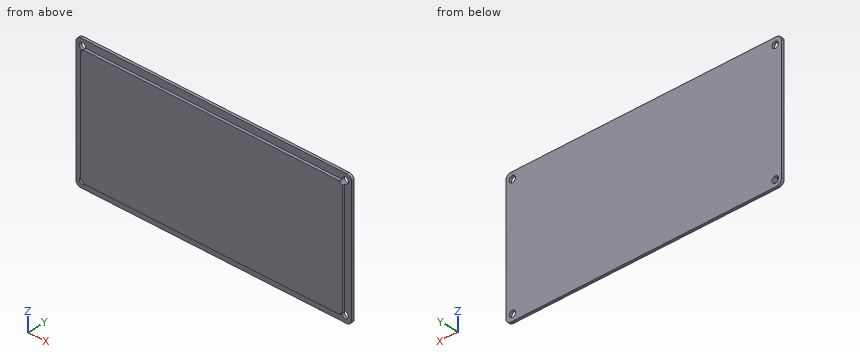
```python
from build123d import *

# Parameters (mm, degrees)
SKETCH2_W           = 127
SKETCH2_H           = 57.15
BOSS_EXTRUDE3_DEPTH = 1.27
SKETCH3_W           = 133.35
SKETCH3_H           = 63.5
BOSS_EXTRUDE4_DEPTH = 1.27
SKETCH4_R           = 1.524
CUT_EXTRUDE1_DEPTH  = 74.892284611
FILLET1_R           = 2.54
SKETCH5_W           = 127
SKETCH5_H           = 57.15
SKETCH5_W_2         = 126.5428
SKETCH5_H_2         = 56.6928
CUT_EXTRUDE2_DEPTH  = 1.27


with BuildPart() as part:
    # Sketch2 → Boss-Extrude3 (new body)
    with BuildSketch(Plane(origin=(0, 0, 0), x_dir=(1, 0, 0), z_dir=(0, 1, 0))):
        Rectangle(SKETCH2_W, SKETCH2_H)
    extrude(amount=BOSS_EXTRUDE3_DEPTH)

    # Sketch3 → Boss-Extrude4 (add)
    with BuildSketch(Plane(origin=(0, 1.27, 0), x_dir=(1, 0, 0), z_dir=(0, 1, 0))):
        Rectangle(SKETCH3_W, SKETCH3_H)
    extrude(amount=BOSS_EXTRUDE4_DEPTH)

    # Sketch4 → Cut-Extrude1 (cut, through all)
    with BuildSketch(Plane(origin=(0, 0, 0), x_dir=(-1, 0, 0), z_dir=(0, -1, 0))):
        with Locations(Location((63.5, -28.575, 0), (0, 0, 90))):
            Circle(SKETCH4_R)
        with Locations(Location((-63.5, -28.575, 0), (0, 0, 90))):
            Circle(SKETCH4_R)
        with Locations(Location((-63.5, 28.575, 0), (0, 0, 90))):
            Circle(SKETCH4_R)
        with Locations(Location((63.5, 28.575, 0), (0, 0, 90))):
            Circle(SKETCH4_R)
    extrude(amount=-CUT_EXTRUDE1_DEPTH, mode=Mode.SUBTRACT)

    # Fillet1
    fillet1_edges = [part.edges().sort_by_distance(p)[0] for p in [
        (66.675, 1.905, 31.75),
        (66.675, 1.905, -31.75),
        (-66.675, 1.905, -31.75),
        (-66.675, 1.905, 31.75),
    ]]
    fillet(fillet1_edges, radius=FILLET1_R)

    # Sketch5 → Cut-Extrude2 (cut)
    with BuildSketch(Plane(origin=(0, 0, 0), x_dir=(-1, 0, 0), z_dir=(0, -1, 0))):
        Rectangle(SKETCH5_W, SKETCH5_H)
        Rectangle(SKETCH5_W_2, SKETCH5_H_2, mode=Mode.SUBTRACT)
    extrude(amount=-CUT_EXTRUDE2_DEPTH, mode=Mode.SUBTRACT)


solid = part.part
```
Geometry: final body of the model. Coordinates: model frame, mm. Round coordinates to 2 decimals unless told otherwise and drop trailing zeros. Order: outer loops, then holes, each group sorted by start corner. A loop starts at its lowest first (then second) coordinate and runs counter-clockwise, first axis right, second up. Notation, with made-up numbers: (8, -33) - (59, -33) arc R22 ccw to (59, 3) - close; hole circle Ø2 at (-16, 61). An arc over 180 degrees is marked (long way). Use CSV: the item, a comma, the result in double quotes. Start each with the question number.
Q1. Section query A-A (z = 20). Return loops of the section in (x, y) (3 decimals).
Q2. First-contact query: pin 1 (1.4 mm diameter, centred on y = 0.5, z = 7.5, fed in from -X); pin 2 (1 mm diameter, centred on x = -30, y = 0.5, fed in from +Z); pin 3 (1 mm diameter, centred on x = 19.5, y = 0.5, fed in from -Z). Flat tips, straight axial feed; report the tip coordinate or a pass-through.
Q3. Section query B-B (y = 0.75). Return loops of the section in (x, z) (3 decimals), and give its area (3 significant figures).
Q4. Material intervals for line 1 along Z through (x, y) = (63.5, 1.3); line 2 along Z through (x, y) = (60, 1.2); line 3 along X through (y, z) = (0.75, -15), sorted ascending. Write a range as from..to.
Result set:
1,outline,"(-66.675, 1.27) - (-63.271, 1.27) - (-63.271, 0) - (63.271, 0) - (63.271, 1.27) - (66.675, 1.27) - (66.675, 2.54) - (-66.675, 2.54) - close"
2,pin 1,"stops at x = -63.27"
2,pin 2,"stops at z = 28.35"
2,pin 3,"stops at z = -28.35"
3,outline,"(-63.271, -27.068) arc R1.524 cw to (-61.993, -28.346) - (61.993, -28.346) arc R1.524 cw to (63.271, -27.068) - (63.271, 27.068) arc R1.524 cw to (61.993, 28.346) - (-61.993, 28.346) arc R1.524 cw to (-63.271, 27.068) - close"
3,area,"7,170 mm2"
4,line 1,"z = -31.75..-30.1, -27.05..27.05, 30.1..31.75"
4,line 2,"z = -28.35..28.35"
4,line 3,"x = -63.27..63.27"
